from build123d import *

# Parameters (mm, degrees)
BOSS_EXTRUDE1_DEPTH     = 19.05
CUT_EXTRUDE1_DEPTH      = 112.559578813
CUT_EXTRUDE1_DEPTH_BACK = 112.559578813
SKETCH2_R               = 1.905
BOSS_EXTRUDE2_START     = 25.4
BOSS_EXTRUDE2_DEPTH     = 8.89
SKETCH5_W               = 19.685
SKETCH5_H               = 10.16
BOSS_EXTRUDE4_DEPTH     = 34.29
CUT_EXTRUDE2_DEPTH      = 123.179346557
CUT_EXTRUDE2_DEPTH_BACK = 123.179346557
SKETCH6_R               = 3.175
CUT_EXTRUDE4_DEPTH      = 123.179346557
CUT_EXTRUDE4_DEPTH_BACK = 123.179346557
SKETCH9_R               = 3.175
FILLET1_R               = 10.16
CUT_EXTRUDE8_DEPTH      = 123.179346557
CUT_EXTRUDE8_DEPTH_BACK = 123.179346557
SKETCH14_R              = 1.905


with BuildPart() as part:
    # Sketch1 → Boss-Extrude1 (new body)
    with BuildSketch(Plane.XY):
        Polygon((44.45, -0.635), (44.45, -10.795), (64.135, -10.795), (64.135, 102.87), (44.45, 102.87), (44.45, 100.33), (44.45, 61.595), (25.4, 61.595), (25.4, 51.435), (51.435, 51.435), (51.435, -0.635), align=None)
    extrude(amount=BOSS_EXTRUDE1_DEPTH)

    # Sketch2 → Cut-Extrude1 (cut, two sides: drawn at the far end of the back side and taken through both)
    with BuildSketch(Plane(origin=(64.135, 0, 0), x_dir=(0, 0, -1), z_dir=(1, 0, 0)).offset(-CUT_EXTRUDE1_DEPTH_BACK)):
        with Locations((-9.525, 91.7575)):
            Circle(SKETCH2_R)
        with Locations((-9.525, 72.7075)):
            Circle(SKETCH2_R)
    extrude(amount=CUT_EXTRUDE1_DEPTH + CUT_EXTRUDE1_DEPTH_BACK, mode=Mode.SUBTRACT)



with BuildPart() as body_2:
    # Sketch3 → Boss-Extrude2 (new body)
    with BuildSketch(Plane.XY.offset(19.05).offset(BOSS_EXTRUDE2_START)):
        with BuildLine():
            Line((25.4, 96.52), (25.4, 102.87))
            Line((25.4, 102.87), (44.45, 102.87))
            Line((44.45, 102.87), (64.135, 102.87))
            Line((64.135, 102.87), (64.135, -10.795))
            Line((64.135, -10.795), (44.45, -10.795))
            Line((44.45, -10.795), (44.45, -0.635))
            Line((44.45, -0.635), (51.435, -0.635))
            Line((51.435, -0.635), (51.435, 51.435))
            Line((51.435, 51.435), (25.4, 51.435))
            Line((25.4, 51.435), (25.4, 61.595))
            Line((25.4, 61.595), (25.4, 67.945))
            ThreePointArc((25.4, 67.945), (39.6875, 82.2325), (25.4, 96.52))
        make_face()
    extrude(amount=BOSS_EXTRUDE2_DEPTH)


with BuildPart() as part_1:
    add(part.part)

    add(body_2.part)  # Boss-Extrude4 merges body 2
    # Sketch5 → Boss-Extrude4 (add)
    with BuildSketch(Plane.XY.offset(53.34)):
        with Locations((54.2925, -5.715)):
            Rectangle(SKETCH5_W, SKETCH5_H)
        with Locations((54.2925, 56.515)):
            Rectangle(SKETCH5_W, SKETCH5_H)
    extrude(amount=-BOSS_EXTRUDE4_DEPTH)

    # Sketch6 → Cut-Extrude2 (cut, two sides: drawn at the far end of the back side and taken through both)
    with BuildSketch(Plane(origin=(64.135, 0, 0), x_dir=(0, 0, -1), z_dir=(1, 0, 0)).offset(-CUT_EXTRUDE2_DEPTH_BACK)):
        with Locations((-14.605, 57.15)):
            Circle(SKETCH6_R)
        with Locations((-4.445, 57.15)):
            Circle(SKETCH6_R)
        with Locations((-14.605, -6.35)):
            Circle(SKETCH6_R)
        with Locations((-4.445, -6.35)):
            Circle(SKETCH6_R)
    extrude(amount=CUT_EXTRUDE2_DEPTH + CUT_EXTRUDE2_DEPTH_BACK, mode=Mode.SUBTRACT)

    # Sketch9 → Cut-Extrude4 (cut, two sides: drawn at the far end of the back side and taken through both)
    with BuildSketch(Plane(origin=(64.135, 0, 0), x_dir=(0, 0, -1), z_dir=(1, 0, 0)).offset(-CUT_EXTRUDE4_DEPTH_BACK)):
        with Locations((-48.895, 57.15)):
            Circle(SKETCH9_R)
        with Locations((-48.895, -6.35)):
            Circle(SKETCH9_R)
    extrude(amount=CUT_EXTRUDE4_DEPTH + CUT_EXTRUDE4_DEPTH_BACK, mode=Mode.SUBTRACT)

    # Fillet1
    # the kernel refuses this fillet: 10.16 mm, written as the material it adds along each edge
    with BuildSketch(Plane(origin=(44.45, 61.595, 19.05), x_dir=(0, 1, 0), z_dir=(1, 0, 0))) as fillet1_piece_1:
        with BuildLine():
            CenterArc((FILLET1_R, FILLET1_R), FILLET1_R, 180, 90)
            Line((0, FILLET1_R), (0, 0))
            Line((0, 0), (FILLET1_R, 0))
        make_face()
    extrude(amount=19.685)
    with BuildSketch(Plane(origin=(64.135, 51.435, 19.05), x_dir=(0, -1, 0), z_dir=(-1, 0, 0)), Plane(origin=(51.435, 51.435, 44.45), x_dir=(0, -1, 0), z_dir=(1, 0, 0))) as fillet1_piece_2:
        with BuildLine():
            CenterArc((FILLET1_R, FILLET1_R), FILLET1_R, 180, 90)
            Line((0, FILLET1_R), (0, 0))
            Line((0, 0), (FILLET1_R, 0))
        make_face()
    extrude(amount=12.7)
    with BuildSketch(Plane(origin=(64.135, 61.595, 44.45), x_dir=(0, 0, -1), z_dir=(-1, 0, 0))) as fillet1_piece_3:
        with BuildLine():
            CenterArc((FILLET1_R, -FILLET1_R), FILLET1_R, 90, 90)
            Line((0, -FILLET1_R), (0, 0))
            Line((0, 0), (FILLET1_R, 0))
        make_face()
    extrude(amount=19.685)
    with BuildSketch(Plane(origin=(64.135, -0.635, 44.45), x_dir=(0, 0, -1), z_dir=(-1, 0, 0)), Plane(origin=(51.435, -0.635, 19.05), x_dir=(0, 0, 1), z_dir=(1, 0, 0))) as fillet1_piece_4:
        with BuildLine():
            CenterArc((FILLET1_R, -FILLET1_R), FILLET1_R, 90, 90)
            Line((0, -FILLET1_R), (0, 0))
            Line((0, 0), (FILLET1_R, 0))
        make_face()
    extrude(amount=12.7)

    # Sketch14 → Cut-Extrude8 (cut, two sides: drawn at the far end of the back side and taken through both)
    with BuildSketch(Plane(origin=(64.135, 0, 0), x_dir=(0, 0, -1), z_dir=(1, 0, 0)).offset(-CUT_EXTRUDE8_DEPTH_BACK)):
        with Locations((-48.895, 99.695)):
            Circle(SKETCH14_R)
    extrude(amount=CUT_EXTRUDE8_DEPTH + CUT_EXTRUDE8_DEPTH_BACK, mode=Mode.SUBTRACT)


solid = part_1.part
The listing builds one solid part. Answer for the finished solid, in the listing's coordinates (mm). A direction names the side the tool comes from. Round coordinates to 2 decimals unless told otherwise and drop trailing zeros. Order: outer loops, then holes, each group sorted by start corner. A loop starts at its lowest first (then second) coordinate and runs counter-clockwise, first axis right, second up. Notation, with made-up numbers: (16.25, 44.25) - (31.25, 44.25) arc R13 cw to (31.25, 54.25) - close; hole circle Ø2 at (80.25, -10). An arc over 180 degrees is marked (long way). Write item = value, one per line. Start each with the question number.
1) Section B-B, the plane z = 31 is taken. Write down the section's boundary in (x, y) (3 decimals).
2) For faces 5 (the flat face through (58, 26, 44.45)), 6 (the flat face through (35, 61.595, 9)), 7 (the flat face through (35, 57, 19.05)), determine the directions among +Z, -Z, +X, -X, +Y, -Y from which every point of the face is accessible in a straight line to the end or side of a thin tool.
3) Given pin 1 (12 mm diameter, centred on y = 3, z = 31, fed in from -X); pin 2 (2.5 mm diameter, centred on x = 50, z = 32.5, fed in from +Y) (3 decimals); pin 3 (2 mm diameter, centred on x = 30, y = 64, fed in from -Z), each flat-ended and moving along its own axis, determine where each tip first touches the part or whether it passes through.
4) Straight lines are drawn through the part: L1, parallel to Z at x = 43.5, y = 57; L2, parallel to Z at x = 49.5, y = 92; L3, parallel to Z at x = 51, y = -6. For each, find the intervals that lie inside material, in ascending order.
5) For a pull along Y with two mould halves and no side action, classify faces 1 (the cylindrical face through (54.4, 64.5, 41.4)), 2 (the flat face through (44.45, -6, 27)), 3 (the cylindrical face through (54.155, 71.017, 8.646)), 4 (the flat face through (49, 51.435, 27)) as released by +Y, released by -Y, zero draft, split by the parting line, or undercut.
6) Section A-A, the plane y = -6.35 is taken. Write down the section's boundary in (x, z) (3 decimals), plus the area to 3 significant figures.
7) Section C-C, the plane y = 33 is taken. Write down the section's boundary in (x, z) (3 decimals).
8) Section D-D, the plane x = 33 is taken. Write down the section's boundary in (y, z) (3 decimals).
Results list:
q1.outline = (44.45, -10.795) - (64.135, -10.795) - (64.135, -0.635) - (44.45, -0.635) - close; (44.45, 51.435) - (64.135, 51.435) - (64.135, 61.595) - (44.45, 61.595) - close
q2.face_5 = +X, -X
q2.face_6 = -Z, -X, +Y
q2.face_7 = -X, +Y, -Y
q3.pin_1 = 44.45
q3.pin_2 = 61.595
q3.pin_3 = 44.45
q4.L1 = 0 to 1.27, 7.62 to 11.43, 17.78 to 19.05, 44.45 to 45.72, 52.07 to 53.34
q4.L2 = 0 to 7.64, 11.41 to 19.05, 44.45 to 53.34
q4.L3 = 0 to 1.29, 7.6 to 11.45, 17.76 to 45.74, 52.05 to 53.34
q5.face_1 = released by +Y
q5.face_2 = zero draft
q5.face_3 = undercut
q5.face_4 = undercut
q6.outline = (44.45, 0) - (64.135, 0) - (64.135, 1.27) - (44.45, 1.27) - close; (44.45, 7.62) - (64.135, 7.62) - (64.135, 11.43) - (44.45, 11.43) - close; (44.45, 17.78) - (64.135, 17.78) - (64.135, 45.72) - (44.45, 45.72) - close; (44.45, 52.07) - (64.135, 52.07) - (64.135, 53.34) - (44.45, 53.34) - close
q6.area = 675 mm^2
q7.outline = (51.435, 0) - (64.135, 0) - (64.135, 19.05) - (51.435, 19.05) - close; (51.435, 44.45) - (64.135, 44.45) - (64.135, 53.34) - (51.435, 53.34) - close
q8.outline = (51.435, 0) - (61.595, 0) - (61.595, 19.05) - (51.435, 19.05) - close; (51.435, 44.45) - (70.134, 44.45) - (70.134, 53.34) - (51.435, 53.34) - close; (94.331, 44.45) - (102.87, 44.45) - (102.87, 53.34) - (94.331, 53.34) - close; hole circle Ø6.35 at (57.15, 4.445); hole circle Ø6.35 at (57.15, 14.605); hole circle Ø6.35 at (57.15, 48.895); hole circle Ø3.81 at (99.695, 48.895)
